Check sheet for the modelled part. Datum: model origin and axes. Units: mm. Round coordinates to 2 decimals unless told otherwise and drop trailing zeros. Order: outer loops, then holes, each group sorted by start corner. A loop starts at its lowest first (then second) coordinate and runs counter-clockwise, first axis right, second up.
Q1. Cross-section at A-A on x = 23. Record the cut outline in (y, z), then the cut area to 3 significant figures.
Q2. Cross-section at D-D on z = 9.5. Record the cut outline in (x, y).
Q3. Cross-section at C-C on z = 1.5. Give the number of separate pieces and of enclosed holes in the cut face, then the cut area to 3 significant figures.
Q4. Scan lines: probe 1 along X at (y, z) = (109, 1.75); probe 2 along Y at (x, z) = (47, 2.05); probe 3 along Z at (x, y) = (3, 98.5). Record each from-to range of solid material in increasing order.
Q5. Depth check by flat-ended pin: P1, Ø18, axis at x = 26.23, y = 33.61, coming from the +Z side; P2, Ø18.5, axis at x = 40.98, y = 19.43, coming from the +Z side; P3, Ø4, axis at x = 41, z = 3, coming from the +Y side; P4, Ø8, axis at x = 46, y = 125, coming from the +Z side. Enter the tip coordinate at first touch or a pass-through.
Q6. Cross-section at B-B on y = 4. Record the cut outline in (x, z).
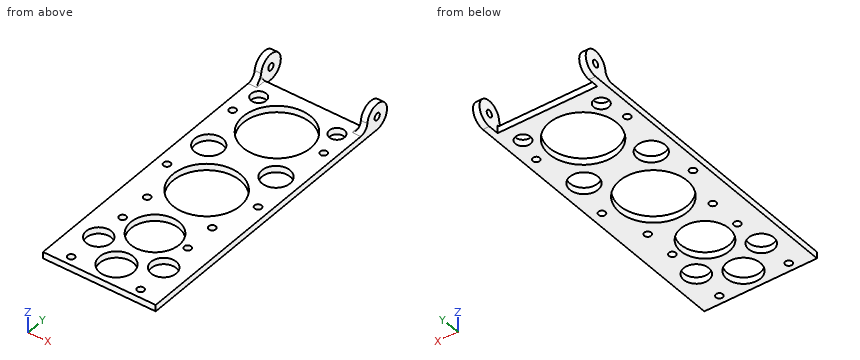
from build123d import *

# Parameters (mm, degrees)
SKETCH003_W   = 46
SKETCH003_H   = 10
PAD003_DEPTH  = 5
SKETCH001_R   = 6
SKETCH001_R_2 = 1.6
PAD001_DEPTH  = 3
SKETCH_W      = 52
SKETCH_H      = 135
SKETCH_R      = 1.6
SKETCH_R_2    = 15.574954
SKETCH_R_3    = 11.186667
SKETCH_R_4    = 6.490241
SKETCH_R_5    = 3.5
SKETCH_R_6    = 7.770751
SKETCH_R_7    = 5.800756
PAD_DEPTH     = 3
SKETCH002_R   = 6
SKETCH002_R_2 = 1.6
PAD002_DEPTH  = 3
FILLET_R      = 4
FILLET001_R   = 4
FILLET002_R   = 1
FILLET003_R   = 1


with BuildPart() as pad003:
    # Sketch003 → Pad003 (new body)
    with BuildSketch(Plane.XY):
        with Locations((26, 135)):
            Rectangle(SKETCH003_W, SKETCH003_H)
    extrude(amount=PAD003_DEPTH)


with BuildPart() as pad001:
    # Sketch001 → Pad001 (new body)
    with BuildSketch(Plane(origin=(0, 135, 0), x_dir=(0, 1, 0), z_dir=(1, 0, 0))):
        with Locations((0, 6)):
            Circle(SKETCH001_R)
        with Locations((0, 6)):
            Circle(SKETCH001_R_2, mode=Mode.SUBTRACT)
    extrude(amount=PAD001_DEPTH)


with BuildPart() as fusion:
    # Sketch → Pad (new body)
    with BuildSketch(Plane.XY):
        with Locations((26, 67.5)):
            Rectangle(SKETCH_W, SKETCH_H)
        with Locations((10, 4)):
            Circle(SKETCH_R, mode=Mode.SUBTRACT)
        with Locations((42, 4)):
            Circle(SKETCH_R, mode=Mode.SUBTRACT)
        with Locations((11, 34)):
            Circle(SKETCH_R, mode=Mode.SUBTRACT)
        with Locations((41, 34)):
            Circle(SKETCH_R, mode=Mode.SUBTRACT)
        with Locations((11, 49)):
            Circle(SKETCH_R, mode=Mode.SUBTRACT)
        with Locations((41, 49)):
            Circle(SKETCH_R, mode=Mode.SUBTRACT)
        with Locations((5, 69)):
            Circle(SKETCH_R, mode=Mode.SUBTRACT)
        with Locations((47, 69)):
            Circle(SKETCH_R, mode=Mode.SUBTRACT)
        with Locations((5, 109)):
            Circle(SKETCH_R, mode=Mode.SUBTRACT)
        with Locations((47, 109)):
            Circle(SKETCH_R, mode=Mode.SUBTRACT)
        with Locations((25.822891, 108.506721)):
            Circle(SKETCH_R_2, mode=Mode.SUBTRACT)
        with Locations((25.87958, 65.548828)):
            Circle(SKETCH_R_2, mode=Mode.SUBTRACT)
        with Locations((26.231028, 33.613125)):
            Circle(SKETCH_R_3, mode=Mode.SUBTRACT)
        with Locations((10.477721, 87.19722)):
            Circle(SKETCH_R_4, mode=Mode.SUBTRACT)
        with Locations((41.522279, 87.19722)):
            Circle(SKETCH_R_4, mode=Mode.SUBTRACT)
        with Locations((7.956594, 121)):
            Circle(SKETCH_R_5, mode=Mode.SUBTRACT)
        with Locations((44.043406, 121)):
            Circle(SKETCH_R_5, mode=Mode.SUBTRACT)
        with Locations((26, 10.44999)):
            Circle(SKETCH_R_6, mode=Mode.SUBTRACT)
        with Locations((11.015624, 19.428881)):
            Circle(SKETCH_R_7, mode=Mode.SUBTRACT)
        with Locations((40.984376, 19.428881)):
            Circle(SKETCH_R_7, mode=Mode.SUBTRACT)
    extrude(amount=PAD_DEPTH)

    # Fusion: union Pad001
    add(pad001.part)


with BuildPart() as fillet003:
    # Sketch002 → Pad002 (new body)
    with BuildSketch(Plane(origin=(49, 135, 0), x_dir=(0, 1, 0), z_dir=(1, 0, 0))):
        with Locations((0, 6)):
            Circle(SKETCH002_R)
        with Locations((0, 6)):
            Circle(SKETCH002_R_2, mode=Mode.SUBTRACT)
    extrude(amount=PAD002_DEPTH)

    # Fusion001: union Fusion
    add(fusion.part)

    # Fillet
    fillet_edges = [fillet003.edges().sort_by_distance(p)[0] for p in [
        (1.5, 129.803848, 3),
    ]]
    fillet(fillet_edges, radius=FILLET_R)

    # Fillet001
    fillet001_edges = [fillet003.edges().sort_by_distance(p)[0] for p in [
        (50.5, 129.803848, 3),
    ]]
    fillet(fillet001_edges, radius=FILLET001_R)

    # Cut: cut Pad003
    add(pad003.part, mode=Mode.SUBTRACT)

    # Fillet002
    fillet002_edges = [fillet003.edges().sort_by_distance(p)[0] for p in [
        (3, 127.426987, 3),
    ]]
    fillet(fillet002_edges, radius=FILLET002_R)

    # Fillet003
    fillet003_edges = [fillet003.edges().sort_by_distance(p)[0] for p in [
        (49, 127.426987, 3),
    ]]
    fillet(fillet003_edges, radius=FILLET003_R)


solid = fillet003.part
Results found:
1. outline: (0, 0) - (3.28, 0) - (3.28, 3) - (0, 3) - close; (17.62, 0) - (22.9, 0) - (22.9, 3) - (17.62, 3) - close; (44.32, 0) - (50.24, 0) - (50.24, 3) - (44.32, 3) - close; (80.86, 0) - (93.19, 0) - (93.19, 3) - (80.86, 3) - close; (123.82, 0) - (130, 0) - (130, 3) - (123.82, 3) - close
1. area: 99.0 mm2
2. outline: (0, 130.13) - (3, 130.13) - (3, 139.87) - (0, 139.87) - close; (49, 130.13) - (52, 130.13) - (52, 139.87) - (49, 139.87) - close
3. separate pieces: 1
3. enclosed holes: 20
3. area: 4,070 mm2
4. probe 1: x = 0 to 3.4, 6.6 to 10.26, 41.39 to 45.4, 48.6 to 52
4. probe 2: y = 0 to 67.4, 70.6 to 83.72, 90.68 to 107.4, 110.6 to 119.13, 122.87 to 130
4. probe 3: z = 0 to 3
5. P1: passes through
5. P2: stops at z = 3
5. P3: stops at y = 130
5. P4: stops at z = 3.96
6. outline: (0, 0) - (8.4, 0) - (8.4, 3) - (0, 3) - close; (11.6, 0) - (21.67, 0) - (21.67, 3) - (11.6, 3) - close; (30.33, 0) - (40.4, 0) - (40.4, 3) - (30.33, 3) - close; (43.6, 0) - (52, 0) - (52, 3) - (43.6, 3) - close
